Could you check a few things on this drawing? It's one solid part, dimensions in mm from its lowest x, y, z. A direction names the side the tool comes from. Round coordinates to 2 decimals unless told otherwise and drop trailing zeros. Order: outer loops, then holes, each group sorted by start corner. A loop starts at its lowest first (then second) coordinate and runs counter-clockwise, first axis right, second up.
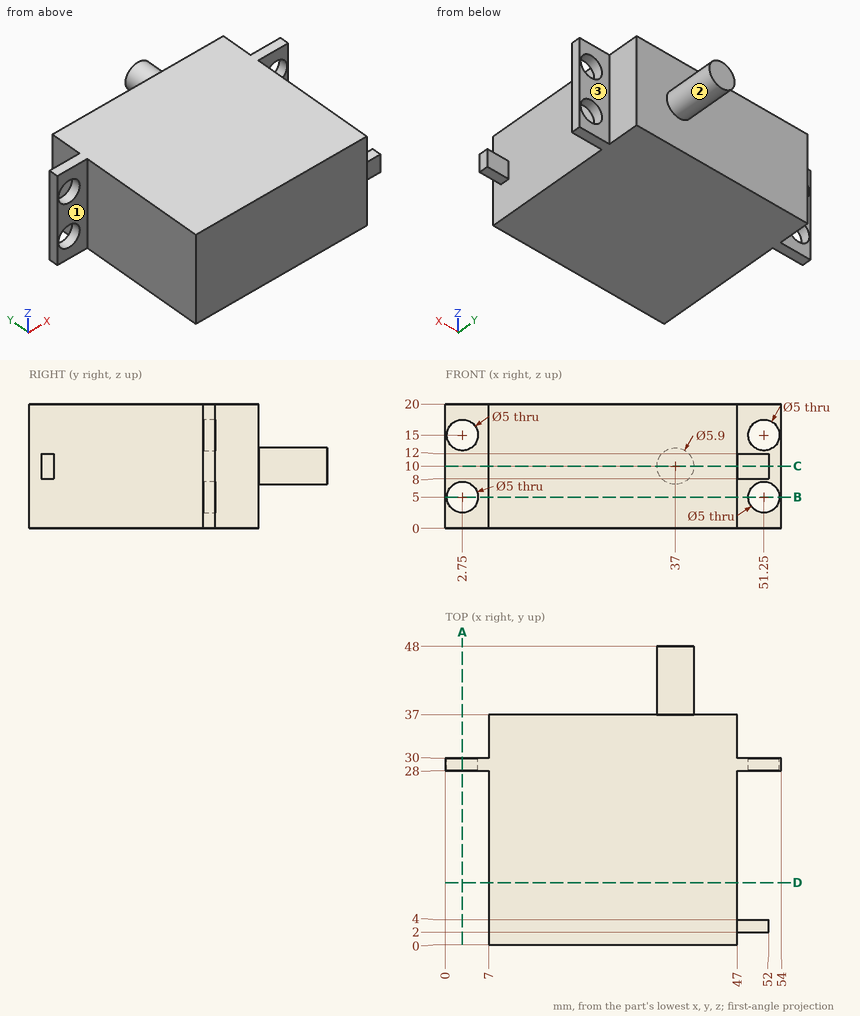
(1) Please list where these lines run through material, in increasing order: probe 1 along X at (y, z) = (29.3, 15); probe 2 along Z at (x, y) = (2, 29); probe 3 along X at (y, z) = (8.5, 7.5).
(2) I'm going to push flat-ended pins straight in: pin 1 Ø3 at (x, z) = (2.75, 15) entering from -Y; pin 2 Ø2 at (y, z) = (32.5, 5.5) entering from +X; pin 3 Ø1 at (x, y) = (50, 3) entering from +Z; pin 4 Ø4 at (y, z) = (38.5, 13) entering from -X. Where does each tip first touch, or does it pass through?
(3) I want a section at B-B, the plane z = 5. List the corners of the cut face in (x, y) for me, plus the area to 3 significant figures.
(4) On a 3-axis mill with a long thin cutter (end or side, diameter ignored), from which of +Z, -Z, +X, -X, +Y, -Y can I reach the whole of each face in a straight line? I mean the marked faces 1, 2 and 3. Say none if no direction works.
(5) I want a section at C-C, the plane z = 10. List the corners of the cut face in (x, y) for me.
(6) I want a section at D-D, the plane y = 10. List the corners of the cut face in (x, z) for me, plus the area to 3 significant figures.
(7) I want a section at A-A, the plane x = 2.75. List the corners of the cut face in (y, z) for me.
Ans:
1. probe 1: x = 0 to 0.25, 5.25 to 48.75, 53.75 to 54
1. probe 2: z = 0 to 2.62, 7.38 to 12.62, 17.38 to 20
1. probe 3: x = 7 to 47
2. pin 1: passes through
2. pin 2: stops at x = 47
2. pin 3: stops at z = 12
2. pin 4: stops at x = 7
3. outline: (0, 28) - (0.25, 28) - (0.25, 30) - (0, 30) - close; (5.25, 28) - (7, 28) - (7, 0) - (47, 0) - (47, 28) - (48.75, 28) - (48.75, 30) - (47, 30) - (47, 37) - (7, 37) - (7, 30) - (5.25, 30) - close; (53.75, 28) - (54, 28) - (54, 30) - (53.75, 30) - close
3. area: 1,490 mm2
4. face 1: +Z, -Z, -X, -Y
4. face 2: +Y
4. face 3: +Z, -Z, +X, +Y
5. outline: (0, 28) - (7, 28) - (7, 0) - (47, 0) - (47, 2) - (52, 2) - (52, 4) - (47, 4) - (47, 28) - (54, 28) - (54, 30) - (47, 30) - (47, 37) - (39.95, 37) - (39.95, 48) - (34.05, 48) - (34.05, 37) - (7, 37) - (7, 30) - (0, 30) - close
6. outline: (7, 0) - (47, 0) - (47, 20) - (7, 20) - close
6. area: 800 mm2
7. outline: (28, 0) - (30, 0) - (30, 2.5) - (28, 2.5) - close; (28, 7.5) - (30, 7.5) - (30, 12.5) - (28, 12.5) - close; (28, 17.5) - (30, 17.5) - (30, 20) - (28, 20) - close
